from build123d import *

# Parameters (mm, degrees)
SKETCH_W     = 20
SKETCH_H     = 20
PAD_DEPTH    = 2.8
SKETCH003_W  = 20
SKETCH003_H  = 12
PAD001_DEPTH = 3.2
POCKET_DEPTH = 10


with BuildPart() as part:
    # Sketch → Pad (new body)
    with BuildSketch(Plane.XY):
        with Locations((-10, 10)):
            Rectangle(SKETCH_W, SKETCH_H)
        with BuildLine():
            ThreePointArc((-12, 17.8), (-13.8, 16), (-12, 14.2))
            Line((-12, 14.2), (-7, 14.2))
            ThreePointArc((-7, 14.2), (-5.2, 16), (-7, 17.8))
            Line((-12, 17.8), (-7, 17.8))
        make_face(mode=Mode.SUBTRACT)
    extrude(amount=PAD_DEPTH)

    # Sketch003 → Pad001 (new body)
    with BuildSketch(Plane.XY.offset(2.8)):
        with Locations((-10, 6)):
            Rectangle(SKETCH003_W, SKETCH003_H)
    extrude(amount=PAD001_DEPTH)

    # Sketch004 → Pocket (cut)
    with BuildSketch(Plane.XY.offset(6)):
        with BuildLine():
            Line((0, 12), (0, 0))
            ThreePointArc((0, 12), (-5.963908, 6), (0, 0))
        make_face()
    extrude(amount=-POCKET_DEPTH, mode=Mode.SUBTRACT)


solid = part.part
CAD build for the part. Positions are in the model's coordinates, mm. A direction names the side the tool comes from. Round coordinates to 2 decimals unless told otherwise and drop trailing zeros. Loops run counter-clockwise (first coordinate to the right, second up) from the corner with the lowest first, then second, coordinate; pieces in that order, holes last. Notation, with made-up numbers: M 53,-8 L 75,-8 A9 ccw 75,-4 Z; hole C -3,3.5 d2. An arc over 180 degrees is marked long. One line per question, with ' | ' between items. Start each with the question number.
Item 1: Wall check: line 1 (Y direction, x = -9.5, z = 1.95); line 2 (Y direction, x = -5, z = 2.4); line 3 (Z direction, x = -19, y = 14). Give the ranges that are in metal, low to high.
Item 2: Cut at C-C, the plane z = 1.3. Write the cut outline in (x, y), plus the area to 3 significant figures.
Item 3: Which spindle directions (+Z, -Z, +X, -X, +Y, -Y) get a long thin tool onto all of the face, cutting with end or side? Do faces 1 (the flat face through (-10, 14.2, 1)), 2 (the flat face through (-10, 12, 4)), 3 (the flat face through (-12, 6, 6)). Say none if no direction does.
Item 4: Cut at D-D, the plane x = -16. Write the cut outline in (y, z), plus the area to 3 significant figures.
Item 5: Pin check, flat tip, straight feed: pin 1 Ø3 at (y, z) = (7.5, 4) entering from +X. Stop position of the tip, or through.
Item 6: Cut at B-B, the plane x = -9.75. Write the cut outline in (y, z).
Item 7: Two-plate mould, pull along X, no slides. Class faces 4 (the flat face through (-10, 18, 2.8)), 5 (the flat face through (-20, 8, 2)), 6 (the cylindrical face through (-13.8, 16, 1.4)), 7 (the cylindrical face through (-5.962, 6.131, 3.042)): pulls with the +X half, pulls with the -X half, needs draft (parallel to the pull), parting line crosses it, or undercut.
Item 8: Cut at A-A, the plane y = 16. Write the cut outline in (x, z), plus the area to 3 significant figures.
Responses:
1) line 1: y = 0 to 14.2, 17.8 to 20 | line 2: y = 0 to 2.74, 9.26 to 20 | line 3: z = 0 to 2.8
2) outline: M -20,0 L 0,0 A6 cw 0,12 L 0,20 L -20,20 Z; hole M -12,14.2 L -7,14.2 A1.8 ccw -7,17.8 L -12,17.8 A1.8 ccw Z | area: 316 mm²
3) face 1: +Z, -Z | face 2: +Z, +X, -X, +Y | face 3: +Z, +X, -X, +Y, -Y
4) outline: M 0,0 L 20,0 L 20,2.8 L 12,2.8 L 12,6 L 0,6 Z | area: 94.4 mm²
5) pin 1: stops at x = -5.16
6) outline: M 0,0 L 14.2,0 L 14.2,2.8 L 12,2.8 L 12,6 L 0,6 Z; M 17.8,0 L 20,0 L 20,2.8 L 17.8,2.8 Z
7) face 4: needs draft | face 5: pulls with the -X half | face 6: undercut | face 7: pulls with the +X half
8) outline: M -20,0 L -13.8,0 L -13.8,2.8 L -20,2.8 Z; M -5.2,0 L 0,0 L 0,2.8 L -5.2,2.8 Z | area: 31.9 mm²
